Design review of the part built by this model. Coordinates are the model's own, in mm. Face numbers are marked on the shaded views. A direction names the side the tool comes from. Round coordinates to 2 decimals unless told otherwise and drop trailing zeros. Order: outer loops, then holes, each group sorted by start corner. A loop starts at its lowest first (then second) coordinate and runs counter-clockwise, first axis right, second up.
from build123d import *

# Parameters (mm, degrees)
RESSALTO_EXTRUS_O1_DEPTH = 8
ESBO_O2_R                = 6
RESSALTO_EXTRUS_O2_DEPTH = 9
ESBO_O3_R                = 8
RESSALTO_EXTRUS_O3_DEPTH = 13
ESBO_O4_R                = 10.5
RESSALTO_EXTRUS_O4_DEPTH = 3.3
RESSALTO_EXTRUS_O6_DEPTH = 25
ESBO_O6_R                = 13.279056191
RESSALTO_EXTRUS_O7_DEPTH = 2
ESBO_O7_R                = 0.6
RESSALTO_EXTRUS_O8_DEPTH = 8


with BuildPart() as part:
    # Esboço1 → Ressalto-extrusão1 (new body)
    with BuildSketch(Plane.XY):
        Polygon((6.639528096, -11.5), (13.279056191, 0), (6.639528096, 11.5), (-6.639528096, 11.5), (-13.279056191, 0), (-6.639528096, -11.5), align=None)
    extrude(amount=RESSALTO_EXTRUS_O1_DEPTH)

    # Esboço2 → Ressalto-extrusão2 (add)
    with BuildSketch(Plane.XY.offset(8)):
        Circle(ESBO_O2_R)
    extrude(amount=RESSALTO_EXTRUS_O2_DEPTH)

    # Esboço3 → Ressalto-extrusão3 (add)
    with BuildSketch(Plane(origin=(0, 0, 0), x_dir=(-1, 0, 0), z_dir=(0, 0, -1))):
        with Locations(Location((0, 0, 0), (0, 0, 180))):
            Circle(ESBO_O3_R)
    extrude(amount=RESSALTO_EXTRUS_O3_DEPTH)

    # Esboço4 → Ressalto-extrusão4 (add)
    with BuildSketch(Plane(origin=(0, 0, -13), x_dir=(-1, 0, 0), z_dir=(0, 0, -1))):
        Circle(ESBO_O4_R)
    extrude(amount=RESSALTO_EXTRUS_O4_DEPTH)

    # Esboço5 → Ressalto-extrusão6 (add)
    with BuildSketch(Plane(origin=(0, 0, -16.3), x_dir=(-1, 0, 0), z_dir=(0, 0, -1))):
        with BuildLine():
            Line((-4.148096191, -2.791647899), (4.148096191, -2.791647899))
            ThreePointArc((4.148096191, -2.791647899), (0, 5), (-4.148096191, -2.791647899))
        make_face()
    extrude(amount=RESSALTO_EXTRUS_O6_DEPTH)

    # Esboço6 → Ressalto-extrusão7 (add)
    with BuildSketch(Plane(origin=(0, 0, 0), x_dir=(-1, 0, 0), z_dir=(0, 0, -1))):
        Circle(ESBO_O6_R)
    extrude(amount=RESSALTO_EXTRUS_O7_DEPTH)

    # Esboço7 → Ressalto-extrusão8 (add)
    with BuildSketch(Plane.XY.offset(17)):
        with Locations((-2.263806511, 3.320249549)):
            Circle(ESBO_O7_R)
        with Locations((2.490187162, 3.320249549)):
            Circle(ESBO_O7_R)
    extrude(amount=RESSALTO_EXTRUS_O8_DEPTH)


solid = part.part
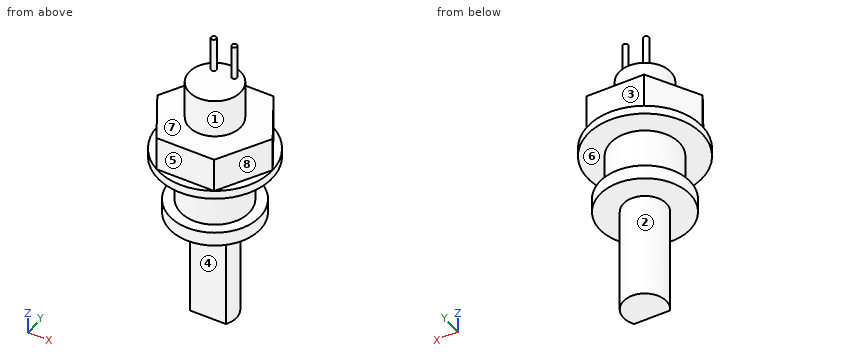
1) Take a section at B-B on z = 16. Give the boundary of the cut face in (x, y), plus the area to 3 significant figures.
Results:
outline: circle Ø12 at (0, 0)
area: 113 mm2
2) Clearance check with flat-ended pins moving along their axes: P1, Ø1, axis at x = -1, y = 4, coming from the +Z side; P2, Ø4, axis at x = -1.5, z = 6, coming from the -Y side; P3, Ø11.5, axis at x = 4.5, y = 0, coming from the +Z side; P4, Ø2.5, axis at x = 1, z = -31.5, coming from the -Y side. State where each tip first meets the part, or that it passes through.
Results:
P1: stops at z = 17
P2: stops at y = -11.5
P3: stops at z = 25
P4: stops at y = -2.79
3) Take a section at D-D on z = -32. Give the boundary of the cut face in (x, y).
Results:
outline: (-4.15, -2.79) - (4.15, -2.79) arc R5 ccw (long way) to start
4) For the marked faces 1, 2, 3, 4 and 5, list the 3-axis set-ups (+Z, -Z, +X, -X, +Y, -Y) from which the entire face can be reached by the end or side of a thin tool; tool diameter is ignored.
Results:
face 1: +Z
face 2: -Z
face 3: +Z, +X, -X, +Y
face 4: -Z, +X, -X, -Y
face 5: +Z, +X, -X, -Y
5) Take a section at A-A on x = 0. Give the boundary of the cut face in (y, z), plus the area to 3 significant figures.
Results:
outline: (-13.28, -2) - (-8, -2) - (-8, -13) - (-10.5, -13) - (-10.5, -16.3) - (-2.79, -16.3) - (-2.79, -41.3) - (5, -41.3) - (5, -16.3) - (10.5, -16.3) - (10.5, -13) - (8, -13) - (8, -2) - (13.28, -2) - (13.28, 0) - (11.5, 0) - (11.5, 8) - (6, 8) - (6, 17) - (-6, 17) - (-6, 8) - (-11.5, 8) - (-11.5, 0) - (-13.28, 0) - close
area: 785 mm2
6) To check wall thickness, follow line 1 along Z through (x, y) = (3, 7.5); line 2 along Z through (x, y) = (-7, 2); line 3 along Z through (x, y) = (-4.25, 3). State the ranges of each line that lie inside material, in increasing order.
Results:
line 1: z = -16.3 to -13, -2 to 8
line 2: z = -16.3 to 8
line 3: z = -16.3 to 17
7) Take a section at C-C on x = 11.25. Give the boundary of the cut face in (y, z), plus the area to 4 significant figures.
Results:
outline: (-7.05, -2) - (7.05, -2) - (7.05, 0) - (3.51, 0) - (3.51, 8) - (-3.51, 8) - (-3.51, 0) - (-7.05, 0) - close
area: 84.45 mm2
8) The part is to be moulded in two halves that separate along Z. For the marked faces 6, 7 and 8, say which applies: released by +Z, released by -Z, zero draft, split by the parting line, or undercut.
Results:
face 6: undercut
face 7: released by +Z
face 8: zero draft
